Could you check a few things on this model? Use its own coordinates, in mm. A direction names the side the tool comes from. Round coordinates to 2 decimals unless told otherwise and drop trailing zeros. Loops run counter-clockwise (first coordinate to the right, second up) from the corner with the lowest first, then second, coordinate; pieces in that order, holes last. Notation, with made-up numbers: M 40,52 L 55,52 A19 ccw 55,60 Z; hole C 34,-23.5 d8. An arc over 180 degrees is marked long. Answer in a Markdown table with one row per item.
```python
from build123d import *

# Parameters (mm, degrees)
SKETCH1_R           = 2
SKETCH1_R_2         = 3
SKETCH1_W           = 3.3
SKETCH1_H           = 9.45
BOSS_EXTRUDE1_DEPTH = 5
SKETCH1_4_W         = 3.3
SKETCH1_4_H         = 9.45
BOSS_EXTRUDE2_DEPTH = 20
CUT_EXTRUDE1_DEPTH  = 3.175
CUT_EXTRUDE2_REACH  = 15
SKETCH2_3_R         = 2.38125


with BuildPart() as part:
    # Sketch1 → Boss-Extrude1 (new body)
    with BuildSketch(Plane.XY):
        with BuildLine():
            Line((-6.5, 1.276325687), (-6.5, -17.71207008))
            ThreePointArc((-6.5, -17.71207008), (0, -24.21207008), (6.5, -17.71207008))
            Line((6.5, -17.71207008), (6.5, 1.276325687))
            Line((6.5, 1.276325687), (-6.5, 1.276325687))
        make_face()
        with Locations((0, -17.71207008)):
            Circle(SKETCH1_R, mode=Mode.SUBTRACT)
        with Locations((0, -5.41207008)):
            Circle(SKETCH1_R_2, mode=Mode.SUBTRACT)
        with BuildLine():
            Line((-6.5, 13.31292992), (-6.5, 1.276325687))
            Line((-6.5, 1.276325687), (6.5, 1.276325687))
            Line((6.5, 1.276325687), (6.5, 13.31292992))
            ThreePointArc((6.5, 13.31292992), (0, 19.81292992), (-6.5, 13.31292992))
        make_face()
        with Locations((0, 8.58792992)):
            Rectangle(SKETCH1_W, SKETCH1_H, mode=Mode.SUBTRACT)
    extrude(amount=BOSS_EXTRUDE1_DEPTH)

    # Sketch1_4 → Boss-Extrude2 (add)
    with BuildSketch(Plane.XY):
        with BuildLine():
            Line((-6.5, 13.31292992), (-6.5, 1.276325687))
            Line((-6.5, 1.276325687), (6.5, 1.276325687))
            Line((6.5, 1.276325687), (6.5, 13.31292992))
            ThreePointArc((6.5, 13.31292992), (0, 19.81292992), (-6.5, 13.31292992))
        make_face()
        with Locations((0, 8.58792992)):
            Rectangle(SKETCH1_4_W, SKETCH1_4_H, mode=Mode.SUBTRACT)
    extrude(amount=BOSS_EXTRUDE2_DEPTH)

    # Sketch2 → Cut-Extrude1 (cut)
    with BuildSketch(Plane.ZY.offset(6.5)):
        Polygon((14.766026472, 8.58792992), (12.383013236, 12.71542992), (7.616986764, 12.71542992), (5.233973528, 8.58792992), (7.616986764, 4.46042992), (12.383013236, 4.46042992), align=None)
    extrude(amount=-CUT_EXTRUDE1_DEPTH, mode=Mode.SUBTRACT)

    # Sketch2_3 → Cut-Extrude2 (cut, up to next)
    with BuildSketch(Plane.ZY.offset(6.5), mode=Mode.PRIVATE) as cut_extrude2_sk1:
        with Locations((10, 8.58792992)):
            Circle(SKETCH2_3_R)
    cut_extrude2_tool1 = extrude(cut_extrude2_sk1.sketch, amount=-CUT_EXTRUDE2_REACH, mode=Mode.PRIVATE) & part.part
    add(cut_extrude2_tool1.solids().sort_by_distance((-6.5, 8.58793, 10))[0], mode=Mode.SUBTRACT)


solid = part.part
```
1) Which directions (+Z, -Z, +X, -X, +Y, -Y) give clear straight access to the entire face, cutting with the end or side of a thin tool? Please do faces 4 (the face through (1.65, 9, 10)), 5 (the face through (-5, 4.46, 10)), 6 (the face through (0, 1.276, 12)).
Computed:
| item | result |
|---|---|
| face 4 | +Z, -Z |
| face 5 | -X |
| face 6 | +Z, +X, -X, -Y |
2) I need wall thicknesses on line 1 (X direction, y = 6.5, z = 13.75); line 2 (Y direction, x = 0, z = 11.75); line 3 (Y direction, x = 0, z = 2). Which ranges of each line are inside material? Lowest first, please.
Computed:
| item | result |
|---|---|
| line 1 | x = -6.5 to -1.65, 1.65 to 6.5 |
| line 2 | y = 1.28 to 3.86, 13.31 to 19.81 |
| line 3 | y = -24.21 to -19.71, -15.71 to -8.41, -2.41 to 3.86, 13.31 to 19.81 |
3) Will these pins go through, and if not, where does the flat tip stop? P1, Ø6, axis at x = -4, y = -12, coming from the -Z side; P2, Ø1.5, axis at x = 2, y = -13.5, coming from the +Z side; P3, Ø1.5, axis at y = 9, z = 10.5, coming from the -X side; P4, Ø4.5, axis at y = 9, z = 11.5, coming from the -X side (3 decimals).
Computed:
| item | result |
|---|---|
| P1 | stops at z = 0 |
| P2 | stops at z = 5 |
| P3 | stops at x = 1.65 |
| P4 | stops at x = -3.325 |
4) I want a section at D-D, the plane y = -9. Please give me the cut outline in (x, z), plus the area to 3 significant figures.
Computed:
| item | result |
|---|---|
| outline | M -6.5,0 L 6.5,0 L 6.5,5 L -6.5,5 Z |
| area | 65.0 mm² |
5) I want a section at C-C, the plane z = 10. Please give me the cut outline in (x, y) (3 decimals).
Computed:
| item | result |
|---|---|
| outline | M -6.5,1.276 L 6.5,1.276 L 6.5,13.313 A6.5 ccw -6.5,13.313 L -6.5,12.715 L -3.325,12.715 L -3.325,10.969 L -1.65,10.969 L -1.65,13.313 L 1.65,13.313 L 1.65,3.863 L -1.65,3.863 L -1.65,6.207 L -3.325,6.207 L -3.325,4.46 L -6.5,4.46 Z |
6) I want a section at B-B, the plane z = 15.5. Please give me the cut outline in (x, y), plus the area to 3 significant figures.
Computed:
| item | result |
|---|---|
| outline | M -6.5,1.28 L 6.5,1.28 L 6.5,13.31 A6.5 ccw -6.5,13.31 Z; hole M -1.65,3.86 L 1.65,3.86 L 1.65,13.31 L -1.65,13.31 Z |
| area | 192 mm² |
7) I want a section at A-A, the plane x = 0. Please give me the cut outline in (y, z), plus the area to 3 significant figures.
Computed:
| item | result |
|---|---|
| outline | M -24.21,0 L -19.71,0 L -19.71,5 L -24.21,5 Z; M -15.71,0 L -8.41,0 L -8.41,5 L -15.71,5 Z; M -2.41,0 L 3.86,0 L 3.86,20 L 1.28,20 L 1.28,5 L -2.41,5 Z; M 13.31,0 L 19.81,0 L 19.81,20 L 13.31,20 Z |
| area | 259 mm² |
8) If we mould it in two halves opening along X, with no side actions, what happens to faces 1 (the face through (-3.325, 10.5, 12.1)), 2 (the face through (-4.93, 6.55, 6.41)), 3 (the face through (-0.434, -19.665, 2.465))? For each: released by +X, released by -X, zero draft, split by the parting line, or undercut.
Computed:
| item | result |
|---|---|
| face 1 | released by -X |
| face 2 | zero draft |
| face 3 | undercut |
